from build123d import *

# Parameters (mm, degrees)
F3_R            = 3.048
F4_DEPTH        = 19.051
F4_COPIES_COUNT = 4


# Not quite as in the source:
# - a pattern or mirror of a feature is missing from the dataset's text; its kind, count and spacing are read off the source's solid


with BuildPart() as f1:
    # F0 (on Right) → F1 (revolve)
    with BuildSketch(Plane.YZ):
        Polygon((-53.848, 19.05), (0, 19.05), (0, 69.85), (-19.05, 69.85), (-19.05, 35.052), (-53.848, 35.052), align=None)
    revolve(axis=Axis((0, -26.924, 0), (0, -1, 0)))

    # F3
    f3_edges = [f1.edges().sort_by_distance(p)[0] for p in [
        (0, -19.05, -69.85),
        (0, 0, -69.85),
        (0, -19.05, -35.052),
        (0, -53.848, -35.052),
    ]]
    fillet(f3_edges, radius=F3_R)

    # F2 (on face) → F4 (cut, through all)
    with BuildSketch(Plane.XZ.offset(19.05)):
        with BuildLine():
            ThreePointArc((-47.498, 0), (-49.2273936601, 4.3557429965), (-53.4735896226, 6.3389523479))
            ThreePointArc((-53.4735896226, 6.3389523479), (-53.848, 0), (-53.4735896226, -6.3389523479))
            ThreePointArc((-53.4735896226, -6.3389523479), (-49.2273936601, -4.3557429965), (-47.498, 0))
        make_face()
        with BuildLine():
            ThreePointArc((-53.4735896226, -6.3389523479), (-53.848, 0), (-53.4735896226, 6.3389523479))
            ThreePointArc((-53.4735896226, 6.3389523479), (-60.198, 0), (-53.4735896226, -6.3389523479))
        make_face()
    f4 = extrude(amount=-F4_DEPTH, mode=Mode.SUBTRACT)

    # F4_copies: F4 ×4 about axis
    f4_copies_axis = Axis((0, 0, 0), (0, 1, 0))
    for i in range(1, F4_COPIES_COUNT):
        add(f4.rotate(f4_copies_axis, i * 360 / F4_COPIES_COUNT), mode=Mode.SUBTRACT)


solid = f1.part
CAD build for the part. Positions are in the model's coordinates, mm. A direction names the side the tool comes from. Round coordinates to 2 decimals unless told otherwise and drop trailing zeros. Order: outer loops, then holes, each group sorted by start corner. A loop starts at its lowest first (then second) coordinate and runs counter-clockwise, first axis right, second up. Notation, with made-up numbers: (30.25, 71.25) -> (37.25, 71.25) arc R17 ccw to (37.25, 85.25) -> close; hole circle Ø2 at (-3.75, 44.5). An arc over 180 degrees is marked (long way). Write item = value, one per line. Start each with the question number.
(1) Cut at A-A, the plane y = -6. List the corners of the cut face in (x, z), then the cut area to 3 significant figures.
(2) Cut at C-C, the plane y = -30.5. List the corners of the cut face in (x, z).
(3) Pin check, flat tips, straight feed: P1, Ø6, axis at x = -10, z = -23, coming from the +Y side; P2, Ø10, axis at x = 38.5, z = 34, coming from the -Y side; P3, Ø4, axis at y = -31.5, z = 15.5, coming from the +X side; P4, Ø12, axis at y = -13, z = -54.5, coming from the +X side. Stop position of each tip, or through.
(4) Which spindle directions (+Z, -Z, +X, -X, +Y, -Y) get a long thin tool onto all of the face, cutting with end or side? Do faces 4 (the flat face through (29, -19.05, 29)), 5 (the flat face through (14, 0, -14)). Say none if no direction does.
(5) Probe line 1 (X direction, y = -26.5, z = 0); line 2 (X direction, y = -13.5, z = -0.5); line 3 (X direction, y = -3.5, z = -4). List the from-to ranges inside material, lowest first. Write a range as [from, to].
(6) Pull direction Z, two halves, no side cores. Call faces 1 (the cylindrical face through (-10.529, -36.65, 33.433)), 2 (the cylindrical face through (11.59, -26.55, -15.12)), 3 (the flat face through (14, -53.848, 14)): released by +Z, released by -Z, zero draft, split by the parting line, or undercut.
(7) Cut at B-B, the plane z = 4.5. State how many separate pieces and enclosed holes the cut face has, then the cut area to 3 significant figures.
Model answer:
q1.outline = circle Ø139.7 at (0, 0); hole circle Ø12.7 at (-53.85, 0); hole circle Ø38.1 at (0, 0); hole circle Ø12.7 at (0, -53.85); hole circle Ø12.7 at (0, 53.85); hole circle Ø12.7 at (53.85, 0)
q1.area = 13,700 mm2
q2.outline = circle Ø70.1 at (0, 0); hole circle Ø38.1 at (0, 0)
q3.P1 = 0
q3.P2 = -19.05
q3.P3 = 32.35
q3.P4 = 50.27
q4.face_4 = -Y
q4.face_5 = +Z, -Z, +X, -X, +Y
q5.line_1 = [-35.05, -19.05], [19.05, 35.05]
q5.line_2 = [-69.85, -60.18], [-47.52, -19.04], [19.04, 47.52], [60.18, 69.85]
q5.line_3 = [-69.74, -58.78], [-48.92, -18.63], [18.63, 48.92], [58.78, 69.74]
q6.face_1 = split by the parting line
q6.face_2 = undercut
q6.face_3 = zero draft
q7.separate_pieces = 4
q7.enclosed_holes = 0
q7.area = 2,730 mm2
